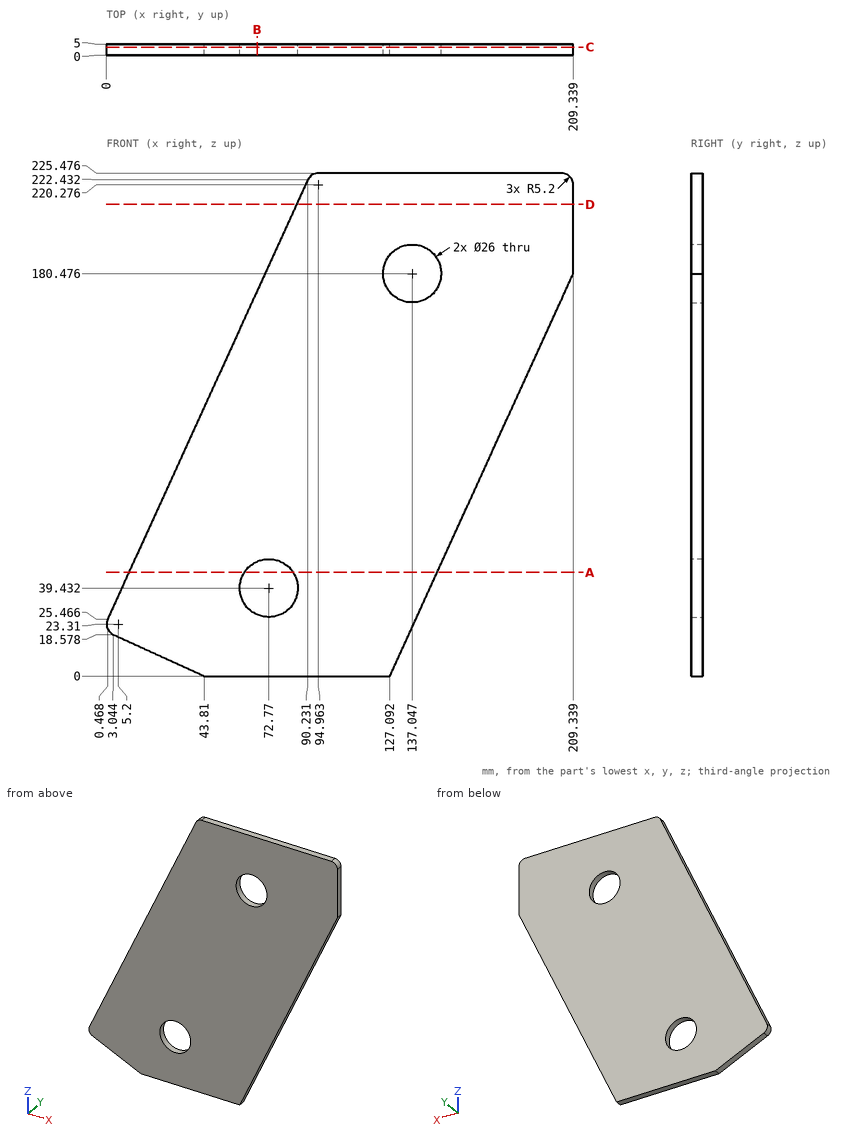
The drawing under review shows one solid part. Ordinate dimensions are in mm from its lowest x, y, z. Round coordinates to 2 decimals unless told otherwise and drop trailing zeros. Order: outer loops, then holes, each group sorted by start corner. A loop starts at its lowest first (then second) coordinate and runs counter-clockwise, first axis right, second up. Notation, with made-up numbers: (45, 89) - (90, 89) arc R14 cw to (90, 114) - close; hole circle Ø10 at (-24, -28.75). An arc over 180 degrees is marked (long way). Return JSON: item names as keys, results as strings.
Q1. For pin 1 Ø15.5 at (x, z) = (72.77, 39.43) entering from +Y, flat-tipped, find the tip position at first contact; note if it passes through.
Computed values:
{"pin 1": "passes through"}
Q2. Consider section C-C on y = 3.65. Write out the cut boundary in (x, z) (1 decimal).
Computed values:
{"outline": "(0.5, 25.5) arc R5.2 ccw to (3, 18.6) - (43.8, 0) - (127.1, 0) - (209.3, 180.5) - (209.3, 220.3) arc R5.2 ccw to (204.1, 225.5) - (95, 225.5) arc R5.2 ccw to (90.2, 222.4) - close; hole circle Ø26 at (72.8, 39.4); hole circle Ø26 at (137, 180.5)"}
Q3. Consider section D-D on z = 211.5. Write out the cut boundary in (x, y).
Computed values:
{"outline": "(85.25, 0) - (209.34, 0) - (209.34, 5) - (85.25, 5) - close"}
Q4. Wall thickness on L1, parallel to Z at x = 131, y = 4.5 (1 decimal); L2, parallel to X at y = 3.75, z = 186 (1 decimal); L3, parallel to Z at x = 140, y = 1.5 (1 decimal): over which ranges is each line inside the solid? List them lowest first. Write a range as [from, to].
Computed values:
{"L1": "z = [8.6, 169], [192, 225.5]", "L2": "x = [73.6, 125.3], [148.8, 209.3]", "L3": "z = [28.3, 167.8], [193.1, 225.5]"}
Q5. Consider section B-B on x = 67.5. Write out the cut boundary in (y, z) (1 decimal).
Computed values:
{"outline": "(0, 0) - (5, 0) - (5, 27.5) - (0, 27.5) - close; (0, 51.3) - (5, 51.3) - (5, 172.6) - (0, 172.6) - close"}
Q6. Consider section A-A on z = 46.5. Write out the cut boundary in (x, y).
Computed values:
{"outline": "(10.05, 0) - (61.86, 0) - (61.86, 5) - (10.05, 5) - close; (83.68, 0) - (148.28, 0) - (148.28, 5) - (83.68, 5) - close"}
